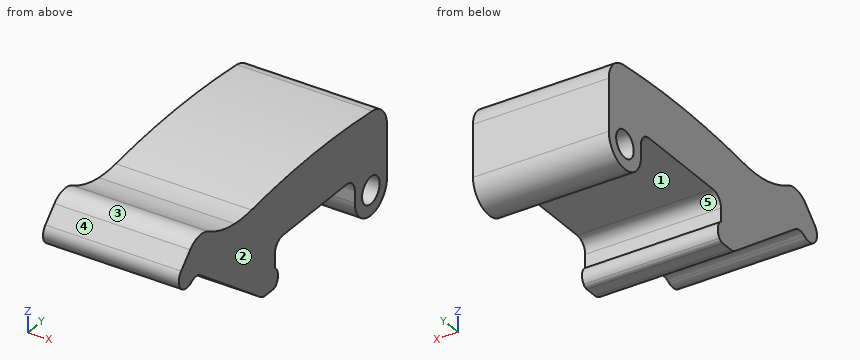
```python
from build123d import *

# Parameters (mm, degrees)
EXTRUDE1_DEPTH              = 8.73125
FILLET1_R                   = 3.175
FILLET2_R                   = 1.5875
FILLET3_R                   = 12.7
FILLET5_R                   = 0.79375
F_29_0_136_DIAMETER_HOLE1_D = 3.4544


with BuildPart() as part:
    # Sketch1 → Extrude1 (new, symmetric)
    with BuildSketch(Plane(origin=(0, 0, 0), x_dir=(0, 0, -1), z_dir=(1, 0, 0))):
        with BuildLine():
            Line((0, 3.175), (-9.525, 3.175))
            ThreePointArc((-9.525, 3.175), (-10.371241591, -10.169917472), (-9.525, -23.514834943))
            ThreePointArc((-9.525, -23.514834943), (-9.557235696, -27.523032937), (-10.655093305, -31.378081441))
            ThreePointArc((-10.655093305, -31.378081441), (-11.542308189, -33.477423108), (-10.675148068, -35.585127786))
            Line((-10.675148068, -35.585127786), (-9.43326403, -36.827011824))
            Line((-9.43326403, -36.827011824), (-8.894448663, -37.365827191))
            ThreePointArc((-8.894448663, -37.365827191), (-6.649384633, -37.365827191), (-6.649384633, -35.120763161))
            Line((-6.649384633, -35.120763161), (-7.1882, -34.581947794))
            Line((-7.1882, -34.581947794), (2.667, -21.336))
            Line((2.667, -21.336), (2.667, -18.923))
            ThreePointArc((2.667, -18.923), (1.397, -18.288), (0.127, -18.923))
            Line((0.127, -18.923), (-3.175, -18.923))
            Line((-3.175, -18.923), (-3.175, -3.175))
            Line((-3.175, -3.175), (0, -3.175))
            ThreePointArc((0, -3.175), (3.175, 0), (0, 3.175))
        make_face()
    extrude(amount=EXTRUDE1_DEPTH, both=True)

    # Fillet1
    fillet1_edges = [part.edges().sort_by_distance(p)[0] for p in [
        (0, 3.175, 9.525),
    ]]
    fillet(fillet1_edges, radius=FILLET1_R)

    # Fillet2
    fillet2_edges = [part.edges().sort_by_distance(p)[0] for p in [
        (0, -3.175, 3.175),
        (0, -34.581947794, 7.1882),
        (0, -21.336, -2.667),
        (0, -18.923, 3.175),
    ]]
    fillet(fillet2_edges, radius=FILLET2_R)

    # Fillet3
    fillet3_edges = [part.edges().sort_by_distance(p)[0] for p in [
        (0, -31.378081441, 10.655093305),
    ]]
    fillet(fillet3_edges, radius=FILLET3_R)

    # Fillet5
    fillet5_edges = [part.edges().sort_by_distance(p)[0] for p in [
        (0, -18.923, -2.667),
    ]]
    fillet(fillet5_edges, radius=FILLET5_R)

    # #29 (0.136) Diameter Hole1 (through all)
    with Locations(Plane(origin=(8.73125, 0, 0), x_dir=(0, 0, -1), z_dir=(1, 0, 0))):
        with Locations((0, 0)):
            Hole(F_29_0_136_DIAMETER_HOLE1_D / 2)


solid = part.part
```
Geometry check sheet. Reference: the model listing, model coordinates, mm. Face numbers are marked on the shaded views. A direction names the side the tool comes from. Give positions to 0.01 mm unless a question says otherwise; leave off trailing zeros. Order: outer loops, then holes, each group sorted by start corner. A loop starts at its lowest first (then second) coordinate and runs counter-clockwise, first axis right, second up. Notation, with made-up numbers: (19.25, 85) -> (51.25, 85) arc R19 ccw to (51.25, 92) -> close; hole circle Ø1 at (-26, 16.25). An arc over 180 degrees is marked (long way). Write each question's results on one line, items separated by ' | '. Start each with the question number.
(1) Sectioned sample at B-B (y = -6.5). Enter the section's corners in (x, z) (3 decimals), plus the area to 3 significant figures.
(2) Gauge pin test, flat ends, axial feed: P1, Ø2, axis at x = 6, y = -32.5, coming from the -Z side; P2, Ø10, axis at x = -6.5, y = -13.5, coming from the +Z side; P3, Ø2, axis at x = 2, y = -27.5, coming from the +Z side. Record the tip position at first contact, or that the pin passes through.
(3) Mould release check, pull along Y, two halves, no side actions. Record for the marked faces 3, 4 and 5: pulls with the +Y half, pulls with the -Y half, needs draft (parallel to the pull), parting line crosses it, or undercut.
(4) Sectioned sample at A-A (y = -1). Enter the section's corners in (x, z), plus the area to 3 significant figures.
(5) Access from +Z, -Z, +X, -X, +Y, -Y to the whole of each face (thin tool, end or side, straight path). Record for the marked faces 1 and 2.
(6) Scan lines: line 1 (Y direction, x = 2, z = 0) (3 decimals); line 2 (Y direction, x = 5, z = -0.25); line 3 (Z direction, x = 2.75, y = -10) (3 decimals). Record each from-to range of solid material in increasing order.
(7) Sectioned sample at C-C (y = -16.5). Enter the section's corners in (x, z) (3 decimals).
Answer below:
1) outline: (-8.731, 3.175) -> (8.731, 3.175) -> (8.731, 10.307) -> (-8.731, 10.307) -> close | area: 125 mm2
2) P1: z = 4.9 | P2: z = 10.37 | P3: z = 9.75
3) face 3: parting line crosses it | face 4: pulls with the -Y half | face 5: undercut
4) outline: (-8.73, -3.01) -> (8.73, -3.01) -> (8.73, -1.41) -> (-8.73, -1.41) -> close; (-8.73, 1.41) -> (8.73, 1.41) -> (8.73, 9.97) -> (-8.73, 9.97) -> close | area: 178 mm2
5) face 1: -Z, +X, -X | face 2: +Z, -Z, +X, +Y, -Y
6) line 1: -24.921 to -18.923, -3.175 to -1.727, 1.727 to 3.175 | line 2: -24.58 to -18.78, -3.17 to -1.71, 1.71 to 3.17 | line 3: 3.175 to 10.371
7) outline: (-8.731, 3.175) -> (8.731, 3.175) -> (8.731, 10.181) -> (-8.731, 10.181) -> close
